CAD build for the part. Positions are in the model's coordinates, mm. A direction names the side the tool comes from. Coordinates: 2 decimals unless noted, no trailing zeros. Order: outer loops, then holes, each group sorted by start corner. A loop starts at its lowest first (then second) coordinate and runs counter-clockwise, first axis right, second up. Notation, with made-up numbers: M -38.75,-3.75 L 9.25,-3.75 A25 ccw 9.25,34.25 Z; hole C 13.25,2 d3. An arc over 180 degrees is marked long. Write item = value, one per line. Start each with the question number.
```python
from build123d import *

# Parameters (mm, degrees)
SKETCH1_W           = 150
SKETCH1_H           = 150
BOSS_EXTRUDE1_DEPTH = 10
SKETCH2_W           = 100
SKETCH2_H           = 100
BOSS_EXTRUDE2_DEPTH = 120
SKETCH3_W           = 42.5
SKETCH3_H           = 42.5
CUT_EXTRUDE1_DEPTH  = 41.5
CHAMFER1_SIZE       = 15
CHAMFER2_SIZE       = 15
SKETCH4_W           = 4.242368117
SKETCH4_H           = 5.545736957
CUT_EXTRUDE2_DEPTH  = 41.5
SKETCH5_W           = 11.091473914
SKETCH5_H           = 11.017090126
CUT_EXTRUDE5_DEPTH  = 24.507631883
CHAMFER3_SIZE       = 5
CHAMFER4_SIZE       = 5
CHAMFER5_SIZE       = 2
SKETCH6_R           = 1.75
CUT_EXTRUDE6_DEPTH  = 10
BOSS_EXTRUDE3_DEPTH = 10
CHAMFER6_SIZE       = 12
SKETCH8_R           = 2.5
CUT_EXTRUDE7_DEPTH  = 10


with BuildPart() as part:
    # Sketch1 → Boss-Extrude1 (new body)
    with BuildSketch(Plane(origin=(0, 0, 0), x_dir=(1, 0, 0), z_dir=(0, 1, 0))):
        Rectangle(SKETCH1_W, SKETCH1_H)
    extrude(amount=BOSS_EXTRUDE1_DEPTH)

    # Sketch2 → Boss-Extrude2 (add)
    with BuildSketch(Plane(origin=(0, 10, 0), x_dir=(1, 0, 0), z_dir=(0, 1, 0))):
        Rectangle(SKETCH2_W, SKETCH2_H)
    extrude(amount=BOSS_EXTRUDE2_DEPTH)

    # Sketch3 → Cut-Extrude1 (cut)
    with BuildSketch(Plane(origin=(0, 130, 0), x_dir=(1, 0, 0), z_dir=(0, 1, 0))):
        Rectangle(SKETCH3_W, SKETCH3_H)
    extrude(amount=-CUT_EXTRUDE1_DEPTH, mode=Mode.SUBTRACT)

    # Chamfer1
    chamfer1_edges = [part.edges().sort_by_distance(p)[0] for p in [
        (75, 5, 75),
        (-75, 5, 75),
        (-75, 5, -75),
        (75, 5, -75),
    ]]
    chamfer(chamfer1_edges, length=CHAMFER1_SIZE)

    # Chamfer2
    chamfer2_edges = [part.edges().sort_by_distance(p)[0] for p in [
        (50, 10, 0),
        (0, 10, -50),
        (50, 70, -50),
        (-50, 10, 0),
        (-50, 70, -50),
    ]]
    chamfer(chamfer2_edges, length=CHAMFER2_SIZE)

    # Sketch4 → Cut-Extrude2 (cut)
    with BuildSketch(Plane(origin=(0, 130, 0), x_dir=(1, 0, 0), z_dir=(0, 1, 0))):
        with Locations((23.371184058, -2.772868478)):
            Rectangle(SKETCH4_W, SKETCH4_H)
        with Locations((23.371184058, 2.772868478)):
            Rectangle(SKETCH4_W, SKETCH4_H)
    extrude(amount=-CUT_EXTRUDE2_DEPTH, mode=Mode.SUBTRACT)

    # Sketch5 → Cut-Extrude5 (cut)
    with BuildSketch(Plane.ZY.offset(-25.492368117)):
        with Locations((0, 94.008545063)):
            Rectangle(SKETCH5_W, SKETCH5_H)
    extrude(amount=-CUT_EXTRUDE5_DEPTH, mode=Mode.SUBTRACT)

    # Chamfer3
    chamfer3_edges = [part.edges().sort_by_distance(p)[0] for p in [
        (50, 94.008545063, 5.545736957),
        (50, 88.5, 0),
        (50, 94.008545063, -5.545736957),
        (50, 99.517090126, 0),
    ]]
    chamfer(chamfer3_edges, length=CHAMFER3_SIZE)

    # Chamfer4
    chamfer4_edges = [part.edges().sort_by_distance(p)[0] for p in [
        (25.492368117, 99.517090126, 0),
    ]]
    chamfer(chamfer4_edges, length=CHAMFER4_SIZE)

    # Chamfer5
    chamfer5_edges = [part.edges().sort_by_distance(p)[0] for p in [
        (21.25, 130, -13.397868478),
        (21.25, 109.25, 5.545736957),
        (21.25, 109.25, -5.545736957),
        (21.25, 130, 13.397868478),
        (0, 130, -21.25),
        (-21.25, 130, 0),
        (0, 130, 21.25),
    ]]
    chamfer(chamfer5_edges, length=CHAMFER5_SIZE)

    # Sketch6 → Cut-Extrude6 (cut)
    with BuildSketch(Plane.XY.offset(50)):
        with Locations((-11, 125.75)):
            Circle(SKETCH6_R)
        with Locations((11, 125.75)):
            Circle(SKETCH6_R)
        with Locations((-11, 14.25)):
            Circle(SKETCH6_R)
        with Locations((11, 14.25)):
            Circle(SKETCH6_R)
    extrude(amount=-CUT_EXTRUDE6_DEPTH, mode=Mode.SUBTRACT)

    # Sketch7 → Boss-Extrude3 (add)
    with BuildSketch(Plane.XY.offset(50)):
        Polygon((54.909019499, 105.514740538), (54.909019499, 20.090980501), (61.512596017, 13.487403983), (61.512596017, 98.91116402), align=None)
    extrude(amount=-BOSS_EXTRUDE3_DEPTH)

    # Chamfer6
    chamfer6_edges = [part.edges().sort_by_distance(p)[0] for p in [
        (58.210807758, 16.789192242, 40),
    ]]
    chamfer(chamfer6_edges, length=CHAMFER6_SIZE)
    # the kernel refuses this chamfer: 12, 8.485281374 mm, written as the material it adds along each edge
    with BuildSketch(Plane(origin=(54.909019499, 20.090980501, 50), x_dir=(-0.7262819568766928, 0.687396915264654, 0), z_dir=(0, 0, -1))) as chamfer6_2_piece_1:
        with BuildLine():
            Line((12.344078342, 0), (5.484140903, 6.49265728))
            Line((5.484140903, 6.49265728), (5.309833233, 6.65763254))
            ThreePointArc((5.309833233, 6.65763254), (2.742070451, 3.24632864), (-0.17430767, 0.16497526))
            Line((-0.17430767, 0.16497526), (0.00659901, -0.23990926))
            ThreePointArc((0.00659901, -0.23990926), (6.173971977, -0.070267795), (12.350677353, -0.23990926))
            Line((12.350677353, -0.23990926), (12.344078342, 0))
        make_face()
    extrude(amount=10)
    with BuildSketch(Plane(origin=(54.909019499, 20.090980501, 40), x_dir=(-0.7262819568766887, 0.6873969152646581, 0), z_dir=(0, 0, -1))) as chamfer6_2_piece_2_section:
        with BuildLine():
            Line((12.344078342, 0), (5.484140903, 6.49265728))
            Line((5.484140903, 6.49265728), (5.309833233, 6.65763254))
            ThreePointArc((5.309833233, 6.65763254), (2.742070451, 3.24632864), (-0.17430767, 0.16497526))
            Line((-0.17430767, 0.16497526), (0.00659901, -0.23990926))
            ThreePointArc((0.00659901, -0.23990926), (6.173971977, -0.070267795), (12.350677353, -0.23990926))
            Line((12.350677353, -0.23990926), (12.344078342, 0))
        make_face()
    chamfer6_2_piece_2 = extrude(amount=42.860195856, mode=Mode.PRIVATE)
    chamfer6_2_piece_2 = split(chamfer6_2_piece_2, bisect_by=Plane(origin=(53.690480503, 27.337708231, 32.262573132), z_dir=(-0.5000000000000001, -0.5000000000000001, 0.7071067811865475)), keep=Keep.TOP, mode=Mode.PRIVATE)
    add(chamfer6_2_piece_2)

    # Sketch8 → Cut-Extrude7 (cut)
    with BuildSketch(Plane(origin=(0, 130, 0), x_dir=(1, 0, 0), z_dir=(0, 1, 0))):
        with Locations(Location((0, 36.625, 0), (0, 0, 270))):
            Circle(SKETCH8_R)
        with Locations(Location((36.625, 0, 0), (0, 0, 270))):
            Circle(SKETCH8_R)
        with Locations(Location((0, -36.625, 0), (0, 0, 270))):
            Circle(SKETCH8_R)
        with Locations(Location((-36.625, 0, 0), (0, 0, 270))):
            Circle(SKETCH8_R)
    extrude(amount=-CUT_EXTRUDE7_DEPTH, mode=Mode.SUBTRACT)


solid = part.part
```
1. 3-axis set-ups, long thin cutter, end or side, ignore diameter. For faces 1 (the flat face through (58, 69, 40)), 2 (the flat face through (-50, 77, 8)), 3 (the flat face through (47.465, 93.861, 8.011)), 4 (the flat face through (25.492, 117, 0)): which of +Z, -Z, +X, -X, +Y, -Y reach the whole face in a straight line?
2. Slice it at A-A (y = 44). Write the cut outline in (x, z).
3. Probe L1, parallel to Y at x = 11, z = 48; L2, parallel to X at y = 125.75, z = 48.25; L3, parallel to X at y = 98, z = -19. List the from-to ranges inside material, lowest first.
4. Flat gauge pins, fed straight in: pin 1 (5 mm diameter, centred on x = -38, y = 110, fed in from -Z); pin 2 (10 mm diameter, centred on y = 74.5, z = 22, fed in from -X); pin 3 (21 mm diameter, centred on x = -6.5, y = 73.5, fed in from -Z). Where does each tip first touch, or does it go through?
5. Mould opens along Z. For faces 5 (the flat face through (-1, 130, 33)), 6 (the flat face through (-1, 5, 75)), 7 (the flat face through (0, 120, -37)), 8 (the flat face through (-47, 16, -47)) say: released by +Z, released by -Z, zero draft, split by the parting line, or undercut.
6. Slice it at C-C (y = 115.5). Write the cut outline in (x, z), plus the area to 3 significant figures.
7. Slice it at D-D (z = 0). Write the cut outline in (x, y) (3 decimals), plus the area to 3 significant figures.
8. Slice it at B-B (z = 46.5). Write the cut outline in (x, y), plus the area to 3 significant figures.
Calculated:
q1.face_1 = -Z, +X, +Y
q1.face_2 = +Z, -Z, -X, +Y
q1.face_3 = +X
q1.face_4 = +Y
q2.outline = M -50,-35 L -35,-50 L 35,-50 L 50,-35 L 50,50 L -50,50 Z; M 54.91,40 L 61.51,40 L 61.51,50 L 54.91,50 Z
q3.L1 = 0 to 12.5, 16 to 124, 127.5 to 130
q3.L2 = -50 to -12.75, -9.25 to 9.25, 12.75 to 50
q3.L3 = -50 to -21.25, 21.25 to 50
q4.pin_1 = -49.5
q4.pin_2 = -50
q4.pin_3 = -50
q5.face_5 = zero draft
q5.face_6 = released by +Z
q5.face_7 = undercut
q5.face_8 = released by -Z
q6.outline = M -50,-35 L -35,-50 L 35,-50 L 50,-35 L 50,50 L -50,50 Z; hole M -21.25,-21.25 L 21.25,-21.25 L 21.25,-7.55 L 23.25,-5.55 L 25.49,-5.55 L 25.49,5.55 L 23.25,5.55 L 21.25,7.55 L 21.25,21.25 L -21.25,21.25 Z
q6.area = 7,920 mm²
q7.outline = M -75,0 L 75,0 L 75,10 L 65,10 L 50,25 L 50,83.5 L 45,88.5 L -21.25,88.5 L -21.25,128 L -23.25,130 L -34.125,130 L -34.125,120 L -39.125,120 L -39.125,130 L -50,130 L -50,25 L -65,10 L -75,10 Z; M 25.492,104.517 L 30.492,99.517 L 45,99.517 L 50,104.517 L 50,130 L 39.125,130 L 39.125,120 L 34.125,120 L 34.125,130 L 25.492,130 Z
q7.area = 11,400 mm²
q8.outline = M -75,0 L 75,0 L 75,10 L 65,10 L 61.51,13.49 L 61.51,98.91 L 54.91,105.51 L 54.91,28.58 L 50,28.58 L 50,130 L -50,130 L -50,25 L -65,10 L -75,10 Z; hole C -11,14.25 d3.5; hole C -11,125.75 d3.5; hole C 11,14.25 d3.5; hole C 11,125.75 d3.5
q8.area = 14,300 mm²
